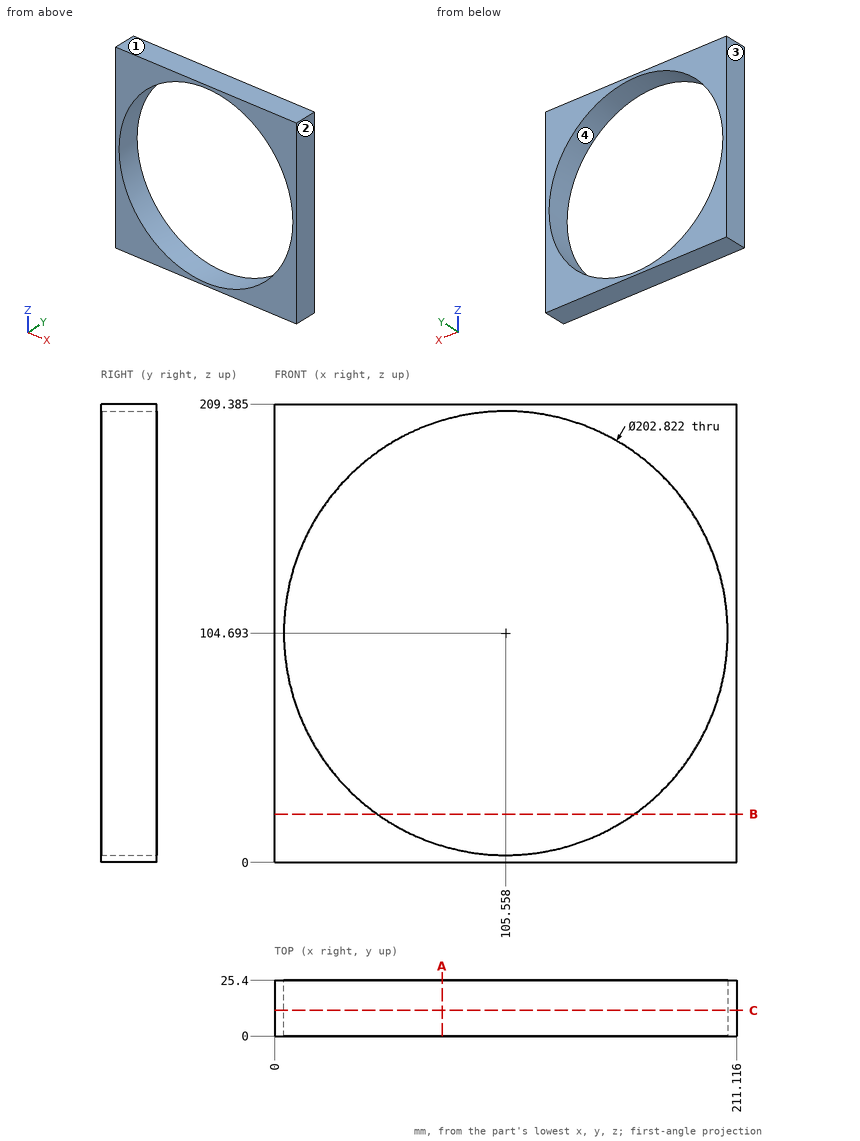
For this review, use the dimensioned drawing (mm, ordinates from the lowest corner) and the shaded views. Round coordinates to 2 decimals unless told otherwise and drop trailing zeros. Order: outer loops, then holes, each group sorted by start corner. A loop starts at its lowest first (then second) coordinate and runs counter-clockwise, first axis right, second up. Notation, with made-up numbers: M -19.75,72 L 5.25,72 A20 ccw 5.25,89 Z; hole C 65.25,81.5 d7. An arc over 180 degrees is marked long. Write each question's results on one line, items separated by ' | '. Start each with the question number.
1. To check wall thickness, follow L1, parallel to X at y = 5.75, z = 107 (1 decimal); L2, parallel to X at y = 8.75, z = 25.5 (1 decimal); L3, parallel to Z at x = 35.5, y = 6.25 (1 decimal). State the ranges of each line that lie inside material, in increasing order. Write a range as [from, to].
2. Draft analysis for pull direction X (two halves, no side actions). For the marked faces 1, 2, 3 and 4, state which applies: pulls with the +X half, pulls with the -X half, needs draft (parallel to the pull), parting line crosses it, or undercut.
3. Add section A-A (x = 76.5). State the section outline as (y, z) points (1 decimal), then the cut area to 3 significant figures.
4. Add section B-B (z = 22). State the section outline as (x, y) points (1 decimal).
5. Add section C-C (y = 11.75). State the section outline as (x, z) points (1 decimal).
Output values:
1) L1: [0, 4.2], [206.9, 211.1] | L2: [0, 42.2], [168.9, 211.1] | L3: [0, 31.4], [178, 209.4]
2) face 1: needs draft | face 2: pulls with the +X half | face 3: pulls with the -X half | face 4: undercut
3) outline: M 0,0 L 25.4,0 L 25.4,7.5 L 0,7.5 Z; M 0,201.9 L 25.4,201.9 L 25.4,209.4 L 0,209.4 Z | area: 383 mm^2
4) outline: M 0,0 L 46.9,0 L 46.9,25.4 L 0,25.4 Z; M 164.3,0 L 211.1,0 L 211.1,25.4 L 164.3,25.4 Z
5) outline: M 0,0 L 211.1,0 L 211.1,209.4 L 0,209.4 Z; hole C 105.6,104.7 d202.8
